For this review, take the finished solid that the model builds, in its own axes (mm). A direction names the side the tool comes from. Give positions to 0.01 mm unless a question says otherwise; leave off trailing zeros. Write each loop counter-clockwise with the first axis right and the second up, starting at its lowest first coordinate (ties: lowest second). Pieces come first, ordered by that corner, then holes. Notation, with made-up numbers: M 40.5,7.5 L 57.5,7.5 A32 cw 57.5,38.5 Z; hole C -10,25.5 d1. An arc over 180 degrees is marked long. One line per item, written item: value. Start each with the question number.
Item 1: Consider section A-A, the plane y = 37. Write out the cut boundary in (x, z), and give its area (3 significant figures).
Item 2: Mouldability with a two-part tool opening along Y and no side actions: class faces 6 (the face through (-22.512, 48.655, -3.944)), 7 (the face through (30.5, -32.9, -3.9)), 8 (the face through (-35.14, -1.273, -3.944)) as released by +Y, released by -Y, zero draft, split by the parting line, or undercut.
Item 3: Consider section B-B, the plane y = -3. Write out the cut boundary in (x, z).
Item 4: Tool access review of faces 1 (the face through (-8.69, 19.67, -3.94)), 2 (the face through (46.17, 4.03, -3.94)), 3 (the face through (-10.87, -31.68, -3.94)), 4 (the face through (-42.568, 19.788, -3.944)), 5 (the face through (-46.34, 4.15, -3.94)): name each direction out of +Z, -Z, +X, -X, +Y, -Y from which nothing blocks a thin tool from reaching the whole face with its end or side.
Item 5: Consider section D-D, the plane y = 25. Write out the cut boundary in (x, z).
Item 6: To check wall thickness, follow probe 1 along Y at (x, z) = (0, -3); probe 2 along X at (y, z) = (4, -6.75); probe 3 along X at (y, z) = (7, -3.5). State the ranges of each line that lie inside material, in increasing order.
Item 7: Consider section C-C, the plane x = -30.5. Write out the cut boundary in (y, z), and give its area (3 significant figures).
Item 8: Clearance check with a flat-ended pin moving along its axis: pin 1 Ø18.5 at (x, y) = (0, 1.78) entering from -Z. State where the tip first meets the part, or that it passes through.
```python
from build123d import *

# Parameters (mm, degrees)
F1_DEPTH = 8


# Not quite as in the source:
# - ends of sketch curves that miss each other by under 0.0002 mm in the source are joined


with BuildPart() as f1:
    # F0 (on Top) → F1 (new body)
    with BuildSketch(Plane.XY):
        with BuildLine():
            ThreePointArc((0.0173106263, 35.2915124556), (-6.457e-07, 35.2914532257), (-0.0173119996, 35.2914272939))
            ThreePointArc((-0.0173119996, 35.2914272939), (-4.7828415657, 36.6814206792), (-8.0865831016, 40.3864729511))
            ThreePointArc((-8.0865831016, 40.3864729511), (-12.5400209066, 46.3598395768), (-18.9133471994, 50.2192344565))
            ThreePointArc((-18.9133471994, 50.2192344565), (-22.5619545404, 48.6311460797), (-26.0784416984, 46.7687064797))
            ThreePointArc((-26.0784416984, 46.7687064797), (-27.0347490245, 39.379546207), (-25.1412558363, 32.173375079))
            ThreePointArc((-25.1412558363, 32.173375079), (-24.3043791298, 27.2803437578), (-26.1889642235, 22.6879091335))
            ThreePointArc((-26.1889642235, 22.6879091335), (-26.1997114341, 22.6743379832), (-26.2105512359, 22.6608403006))
            ThreePointArc((-26.2105512359, 22.6608403006), (-30.268483933, 19.8015929347), (-35.2250588486, 19.5286856632))
            ThreePointArc((-35.2250588486, 19.5286856632), (-42.6718988891, 19.7711813344), (-49.6630001039, 17.1946071711))
            ThreePointArc((-49.6630001039, 17.1946071711), (-50.6962513252, 13.3518540399), (-51.4326312922, 9.4413418946))
            ThreePointArc((-51.4326312922, 9.4413418946), (-46.2518013791, 4.086604184), (-39.4372158458, 1.0740226787))
            ThreePointArc((-39.4372158458, 1.0740226787), (-35.0899055663, -1.3224359394), (-32.6744151986, -5.6592003729))
            ThreePointArc((-32.6744151986, -5.6592003729), (-32.6705053342, -5.676064432), (-32.6666279149, -5.6929359805))
            ThreePointArc((-32.6666279149, -5.6929359805), (-32.9613409881, -10.648285961), (-35.8383477489, -14.6936473148))
            ThreePointArc((-35.8383477489, -14.6936473148), (-40.6709671644, -20.3646275254), (-43.0154005889, -27.4369580526))
            ThreePointArc((-43.0154005889, -27.4369580526), (-40.655237183, -30.6407045779), (-38.0570010523, -33.6545940487))
            ThreePointArc((-38.0570010523, -33.6545940487), (-30.6403035701, -32.942681267), (-24.0361481426, -29.4931378216))
            ThreePointArc((-24.0361481426, -29.4931378216), (-19.4520178261, -27.5884419734), (-14.5553656824, -28.4038640421))
            ThreePointArc((-14.5553656824, -28.4038640421), (-14.539742708, -28.4113209434), (-14.5241712519, -28.4188855039))
            ThreePointArc((-14.5241712519, -28.4188855039), (-10.8336363316, -31.7388351981), (-9.46463, -36.510411))
            ThreePointArc((-9.46463, -36.510411), (-8.0439677673, -43.8245030704), (-3.9763277521, -50.0669807595))
            ThreePointArc((-3.9763277521, -50.0669807595), (-4.985e-07, -50.219235), (3.9763270429, -50.066981559))
            ThreePointArc((3.9763270429, -50.066981559), (8.0439676368, -43.8245033926), (9.4646296494, -36.5104109994))
            ThreePointArc((9.4646296494, -36.5104109994), (10.8336355705, -31.738834816), (14.5241710621, -28.4188851093))
            ThreePointArc((14.5241710621, -28.4188851093), (14.5397421135, -28.4113207469), (14.555327686, -28.4037863488))
            ThreePointArc((14.555327686, -28.4037863488), (19.4520168261, -27.5884419734), (24.0361467636, -29.4931382964))
            ThreePointArc((24.0361467636, -29.4931382964), (30.6403030472, -32.9426814086), (38.0570009358, -33.6545933411))
            ThreePointArc((38.0570009358, -33.6545933411), (40.655237183, -30.6407045779), (43.0154002031, -27.436958138))
            ThreePointArc((43.0154002031, -27.436958138), (40.6709661644, -20.3646275254), (35.8383467951, -14.6936472574))
            ThreePointArc((35.8383467951, -14.6936472574), (32.9613408944, -10.6482856952), (32.6667108543, -5.6929547524))
            ThreePointArc((32.6667108543, -5.6929547524), (32.6705043598, -5.6760643215), (32.67441425, -5.659200152))
            ThreePointArc((32.67441425, -5.659200152), (35.0899046467, -1.3224358594), (39.4372149344, 1.0740222872))
            ThreePointArc((39.4372149344, 1.0740222872), (46.2518003791, 4.086604184), (51.4326310926, 9.4413419398))
            ThreePointArc((51.4326310926, 9.4413419398), (50.6962513088, 13.3518541117), (49.6629990471, 17.1946070146))
            ThreePointArc((49.6629990471, 17.1946070146), (42.6718983702, 19.7711812567), (35.2250588084, 19.5286858355))
            ThreePointArc((35.2250588084, 19.5286858355), (30.2684833934, 19.8015927747), (26.2105502359, 22.6608403006))
            ThreePointArc((26.2105502359, 22.6608403006), (26.1997106027, 22.6743373459), (26.1889636103, 22.687908644))
            ThreePointArc((26.1889636103, 22.687908644), (24.3043781641, 27.2803434477), (25.1412552893, 32.1733748607))
            ThreePointArc((25.1412552893, 32.1733748607), (27.0347490207, 39.3795461477), (26.0784413783, 46.768707126))
            ThreePointArc((26.0784413783, 46.768707126), (22.5619541507, 48.6311462674), (18.9133467528, 50.2192343669))
            ThreePointArc((18.9133467528, 50.2192343669), (12.5400199066, 46.3598395768), (8.0865821819, 40.3864729126))
            ThreePointArc((8.0865821819, 40.3864729126), (4.7828405657, 36.6814206792), (0.0173106263, 35.2915124556))
        make_face()
        with BuildLine():
            Line((-10.813517, 12.711431), (-13.133307, 17.528522))
            Line((-13.133307, 17.528522), (-4.123619, 21.867361))
            Line((-4.123619, 21.867361), (-1.803829, 17.050271))
            ThreePointArc((-1.803829, 17.050271), (6.6712619157, -12.0722441106), (-10.813517, 12.711431))
        make_face(mode=Mode.SUBTRACT)
    extrude(amount=-F1_DEPTH)


solid = f1.part
```
Model answer:
1. outline: M -26.73,-8 L -5.25,-8 L -5.25,0 L -26.73,0 Z; M 5.25,-8 L 26.73,-8 L 26.73,0 L 5.25,0 Z
1. area: 344 mm2
2. face 6: released by +Y
2. face 7: released by -Y
2. face 8: undercut
3. outline: M -33.76,-8 L -14.61,-8 L -14.61,0 L -33.76,0 Z; M 14.61,-8 L 33.76,-8 L 33.76,0 L 14.61,0 Z
4. face 1: +Z, -Z
4. face 2: +Z, -Z, +X
4. face 3: +Z, -Z, -Y
4. face 4: +Z, -Z, +Y
4. face 5: +Z, -Z, -X
5. outline: M -24.86,-8 L 24.86,-8 L 24.86,0 L -24.86,0 Z
6. probe 1: y = -50.22 to -13.59, 17.16 to 35.29
6. probe 2: x = -46.13 to -15.21, 15.21 to 46.13
6. probe 3: x = -49.56 to -14.46, 14.46 to 49.56
7. outline: M -32.9,-8 L 19.72,-8 L 19.72,0 L -32.9,0 Z
7. area: 421 mm2
8. pin 1: passes through
